The model under review builds one solid part; all positions refer to its coordinate system, in mm. A direction names the side the tool comes from. Give positions to 0.01 mm unless a question says otherwise; leave off trailing zeros. Order: outer loops, then holes, each group sorted by start corner. A loop starts at its lowest first (then second) coordinate and runs counter-clockwise, first axis right, second up. Notation, with made-up numbers: (33.25, -29.75) -> (51.25, -29.75) arc R10 ccw to (51.25, -14.75) -> close; hole circle Ø6 at (-10.75, 66). An arc over 180 degrees is marked (long way). Use one line per item in the form item = value.
```python
from build123d import *

# Parameters (mm, degrees)
SKETCH3_R           = 8.5
SKETCH1_R           = 8
SKETCH4_R           = 2.5
BOSS_EXTRUDE1_DEPTH = 17
SKETCH5_R           = 4.5
CUT_EXTRUDE1_DEPTH  = 2
SKETCH6_R           = 1
CUT_EXTRUDE4_DEPTH  = 6
SKETCH8_R           = 2
CUT_EXTRUDE5_DEPTH  = 1
FILLET1_R           = 1
CHAMFER1_SIZE       = 0.4
FILLET2_R           = 1


with BuildPart() as part:
    # Sketch3 → Loft1 section 0
    with BuildSketch(Plane(origin=(0, 6, 0), x_dir=(1, 0, 0), z_dir=(0, 1, 0))):
        Circle(SKETCH3_R)
    # Sketch1 → Loft1 section 1
    with BuildSketch(Plane(origin=(0, 0, 0), x_dir=(1, 0, 0), z_dir=(0, 1, 0))):
        Circle(SKETCH1_R)
    loft()

    # Sketch4 → Boss-Extrude1 (add)
    with BuildSketch(Plane(origin=(0, 6, 0), x_dir=(1, 0, 0), z_dir=(0, 1, 0))):
        with Locations(Location((0, 0, 0), (0, 0, 270))):
            Circle(SKETCH4_R)
    extrude(amount=BOSS_EXTRUDE1_DEPTH)

    # Sketch5 → Cut-Extrude1 (cut)
    with BuildSketch(Plane.XZ):
        with Locations(Location((0, 0, 0), (0, 0, 270))):
            Circle(SKETCH5_R)
    extrude(amount=-CUT_EXTRUDE1_DEPTH, mode=Mode.SUBTRACT)

    # Sketch6 → Cut-Extrude4 (cut)
    with BuildSketch(Plane.XZ):
        with Locations(Location((0, 6.25, 0), (0, 0, 270))):
            Circle(SKETCH6_R)
        with Locations(Location((6.25, 0, 0), (0, 0, 270))):
            Circle(SKETCH6_R)
        with Locations(Location((0, -6.25, 0), (0, 0, 270))):
            Circle(SKETCH6_R)
        with Locations(Location((-6.25, 0, 0), (0, 0, 270))):
            Circle(SKETCH6_R)
    extrude(amount=-CUT_EXTRUDE4_DEPTH, mode=Mode.SUBTRACT)

    # Sketch8 → Cut-Extrude5 (cut)
    with BuildSketch(Plane.XZ.offset(-2)):
        with Locations(Location((0, 0, 0), (0, 0, 270))):
            Circle(SKETCH8_R)
    extrude(amount=-CUT_EXTRUDE5_DEPTH, mode=Mode.SUBTRACT)

    # Fillet1
    fillet1_edges = [part.edges().sort_by_distance(p)[0] for p in [
        (0, 2, 2),
    ]]
    fillet(fillet1_edges, radius=FILLET1_R - 0.0001)  # a hair under: the kernel refuses the full size

    # Chamfer1
    chamfer1_edges = [part.edges().sort_by_distance(p)[0] for p in [
        (0, 23, -2.5),
    ]]
    chamfer(chamfer1_edges, length=CHAMFER1_SIZE)

    # Fillet2
    fillet2_edges = [part.edges().sort_by_distance(p)[0] for p in [
        (0, 6, 7.25),
        (6.25, 6, 1),
        (0, 6, -5.25),
        (-6.25, 6, 1),
    ]]
    fillet(fillet2_edges, radius=FILLET2_R)


solid = part.part
```
1. For L1, parallel to X at y = 2.4, z = 0; L2, parallel to X at y = 1.9, z = 0; L3, parallel to Y at x = 4.25, z = 6.25, list the stretches that pass through material, from the lowest coordinate up.
Values:
L1 = -8.2 to -7.25, -5.25 to -2.2, 2.2 to 5.25, 7.25 to 8.2
L2 = -8.16 to -7.25, -5.25 to -4.5, 4.5 to 5.25, 7.25 to 8.16
L3 = 0 to 6
2. Tool access review of faces 1 (the face through (0, 3, 0)), 2 (the face through (7.24, 2.46, 0.13)), 3 (the face through (2, 6, 2)): name each direction out of +Z, -Z, +X, -X, +Y, -Y from which nothing blocks a thin tool from reaching the whole face with its end or side.
Values:
face_1 = -Y
face_2 = +Y, -Y
face_3 = +Y
3. For pin 1 Ø2.5 at (x, z) = (-6.25, 0) entering from -Y; pin 2 Ø6 at (x, y) = (4.5, 6) entering from -Z; pin 3 Ø2.5 at (x, z) = (0, -6.25) entering from +Y; pin 4 Ø8 at (y, z) = (14, 4.5) entering from -X, all flat-tipped, find the tip position at first contact; note any pin that passes through.
Values:
pin_1 = 0
pin_2 = -8.37
pin_3 = 5.66
pin_4 = -2.45
4. Add section B-B on y = 14.5. Give the boundary of the cut face in (x, z), then the cut area to 3 significant figures.
Values:
outline = circle Ø5 at (0, 0)
area = 19.6 mm^2
5. The part is to be moulded in two halves that separate along X. For faces 4 (the face through (0, 23, 0)), 5 (the face through (-2.44, 14.18, -0.54)), 6 (the face through (-0.61, 2.46, -5.46)), say which applies: +X half, -X half, draft (parallel to the pull), parting line (faces both ways), or undercut.
Values:
face_4 = draft
face_5 = parting line
face_6 = undercut
6. Add section A-A on x = 0. Count the separate pieces of the cut face and the enclosed holes in it, then the cut area to 3 significant figures.
Values:
separate_pieces = 3
enclosed_holes = 0
area = 137 mm^2
